Read the model definition and answer for the solid it produces. Units are mm, in the model's axes. A direction names the side the tool comes from. Coordinates: 2 decimals unless noted, no trailing zeros. Write each loop counter-clockwise with the first axis right and the second up, starting at its lowest first coordinate (ties: lowest second). Pieces come first, ordered by that corner, then holes.
Item 1: Section C-C (y = -15.75) is taken. Give the vertices of the cut face in (x, z).
Item 2: A tool of negligible diameter and unlimited length cuts with its end or side. For faces 1 (the face through (-4.483, -13, 3)), 2 (the face through (-9.82, -5.13, 6.9)), from which of +Z, -Z, +X, -X, +Y, -Y can it reach the whole face along a straight path? Write none if from no direction.
Item 3: Straight lines are drawn through the part: probe 1 along X at (y, z) = (-6.35, 8.25); probe 2 along X at (y, z) = (-19.05, 5.75); probe 3 along X at (y, z) = (-11.75, 2.5). For each, find the intervals that lie inside material, in ascending order.
Item 4: This flat-tipped pin is pushed along its axis until it touches: P1, Ø1, axis at x = 5.5, z = 8, coming from the +Y side. Where does it stop, or does it pass through?
Item 5: Section A-A (z = 2) is taken. Give the vertices of the cut face in (x, y).
Item 6: Section B-B (z = 8.25) is taken. Give the vertices of the cut face in (x, y), then the cut area to 3 significant figures.
Item 7: Determine the mould class of faces 3 (the face through (0, -13, 7)), 4 (the face through (9, -13, 0)), 5 (the face through (5.517, -13, 4)), 6 (the face through (-11.983, -13, 7)) for opening direction X: released by +X, released by -X, zero draft, split by the parting line, or undercut.
Item 8: Section D-D (x = 10) is taken. Give the vertices of the cut face in (y, z), then the cut area to 3 significant figures.
from build123d import *

# Parameters (mm, degrees)
F1_DEPTH = 25.4
F2_R     = 2
F3_DEPTH = 14.001


with BuildPart() as f1:
    # F0 (on Front) → F1 (new body)
    with BuildSketch(Plane.XZ):
        Polygon((-11.982759, 14), (-11.982759, 0), (-4.482759, 0), (-4.482759, 7), (5.517241, 7), (5.517241, 0), (13.017241, 0), (13.017241, 14), align=None)
    extrude(amount=F1_DEPTH)

    # F2 (on face) → F3 (cut, through all)
    with BuildSketch(Plane(origin=(0, 0, 0), x_dir=(1, 0, 0), z_dir=(0, 0, -1))):
        with BuildLine():
            ThreePointArc((9.267241, 21.05), (7.853028, 17.635786), (11.267241, 19.05))
            ThreePointArc((11.267241, 19.05), (10.681455, 20.464214), (9.267241, 21.05))
        make_face()
        with BuildLine():
            ThreePointArc((9.267241, 4.35), (10.681455, 4.935786), (11.267241, 6.35))
            ThreePointArc((11.267241, 6.35), (7.853028, 7.764214), (9.267241, 4.35))
        make_face()
        with Locations((-8.232759, 6.35)):
            Circle(F2_R)
        with Locations((-8.232759, 19.05)):
            Circle(F2_R)
    extrude(amount=-F3_DEPTH, mode=Mode.SUBTRACT)


solid = f1.part
Established:
1. outline: (-11.98, 0) - (-4.48, 0) - (-4.48, 7) - (5.52, 7) - (5.52, 0) - (13.02, 0) - (13.02, 14) - (-11.98, 14) - close
2. face 1: -Z, +Y, -Y
2. face 2: +Z, -Z
3. probe 1: x = -11.98 to -10.23, -6.23 to 7.27, 11.27 to 13.02
3. probe 2: x = -11.98 to -10.23, -6.23 to -4.48, 5.52 to 7.27, 11.27 to 13.02
3. probe 3: x = -11.98 to -4.48, 5.52 to 13.02
4. P1: stops at y = 0
5. outline: (-11.98, -25.4) - (-4.48, -25.4) - (-4.48, 0) - (-11.98, 0) - close; (5.52, -25.4) - (13.02, -25.4) - (13.02, 0) - (5.52, 0) - close; hole circle Ø4 at (-8.23, -19.05); hole circle Ø4 at (-8.23, -6.35); hole (9.27, -21.05) arc R2 ccw to (11.27, -19.05) arc R2 ccw (long way) to start; hole (9.27, -4.35) arc R2 ccw (long way) to (11.27, -6.35) arc R2 ccw to start
6. outline: (-11.98, -25.4) - (13.02, -25.4) - (13.02, 0) - (-11.98, 0) - close; hole circle Ø4 at (-8.23, -19.05); hole circle Ø4 at (-8.23, -6.35); hole (9.27, -21.05) arc R2 ccw to (11.27, -19.05) arc R2 ccw (long way) to start; hole (9.27, -4.35) arc R2 ccw (long way) to (11.27, -6.35) arc R2 ccw to start
6. area: 585 mm2
7. face 3: undercut
7. face 4: zero draft
7. face 5: undercut
7. face 6: released by -X
8. outline: (-25.4, 0) - (-20.91, 0) - (-20.91, 14) - (-25.4, 14) - close; (-17.19, 0) - (-8.21, 0) - (-8.21, 14) - (-17.19, 14) - close; (-4.49, 0) - (0, 0) - (0, 14) - (-4.49, 14) - close
8. area: 251 mm2
